CAD build for the part. Positions are in the model's coordinates, mm. Face numbers are marked on the shaded views. Give positions to 0.01 mm unless a question says otherwise; leave off trailing zeros. Loops run counter-clockwise (first coordinate to the right, second up) from the corner with the lowest first, then second, coordinate; pieces in that order, holes last. Notation, with made-up numbers: M 15,29 L 26,29 A14 ccw 26,52 Z; hole C 31,56 d6. An arc over 180 degrees is marked long. Answer as CSV lines item,"result".
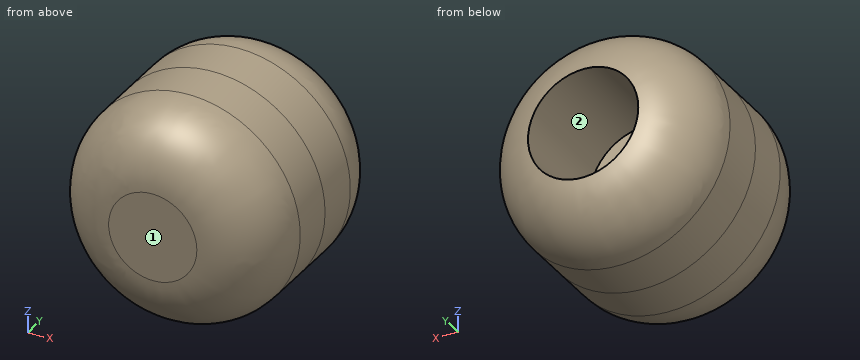
from build123d import *

# Parameters (mm, degrees)
F0_R     = 6.35
F1_DEPTH = 6.35
F2_R     = 6.35
F2_R_2   = 3.175
F3_DEPTH = 6.35


# Not quite as in the source:
# - a fillet or chamfer that OpenCascade refuses, or shapes differently, is made with other operations: its cross-section is extruded or revolved along the edge and cut away or added


with BuildPart() as f1:
    # F0 (on Front) → F1 (new body)
    with BuildSketch(Plane.XZ):
        Circle(F0_R)
    extrude(amount=F1_DEPTH)

    # F2 (on face) → F3 (join)
    with BuildSketch(Plane(origin=(0, 0, 0), x_dir=(-1, 0, 0), z_dir=(0, 1, 0))):
        Circle(F2_R)
        Circle(F2_R_2, mode=Mode.SUBTRACT)
    extrude(amount=F3_DEPTH)

    # F4: fillet of radius 3.81 on 2 edges, made by hand

    # F4_s1 → F4_t2 (revolve, cut)
    with BuildSketch(Plane.XY):
        with BuildLine():
            ThreePointArc((-6.35, 2.5932893377), (-5.4499355663, 5.0526337626), (-3.175, 6.35))
            Line((-3.175, 6.35), (-6.35, 6.35))
            Line((-6.35, 6.35), (-6.35, 2.5932893377))
        make_face()
    revolve(axis=Axis((0, 6.35, 0), (0, 1, 0)), mode=Mode.SUBTRACT)

    # F4_s3 → F4_t4 (revolve, cut)
    with BuildSketch(Plane.XY):
        with BuildLine():
            ThreePointArc((6.35, -2.54), (5.2340768363, -5.2340768363), (2.54, -6.35))
            Line((2.54, -6.35), (6.35, -6.35))
            Line((6.35, -6.35), (6.35, -2.54))
        make_face()
    revolve(axis=Axis((0, -6.35, 0), (0, -1, 0)), mode=Mode.SUBTRACT)


solid = f1.part
1) Band-saw the part on A-A on y = 1.75. Give the cut face in (x, z) (3 decimals), and give its area (3 significant figures).
Answer below:
outline,"C 0,0 d12.7; hole C 0,0 d6.35"
area,"95.0 mm^2"
2) Drill centre lines: line 1 (Z direction, x = 0, y = 1.75) (3 decimals); line 2 (Z direction, x = 5.5, y = 0.75); line 3 (Z direction, x = -2.25, y = 5.25). Where is each one in solid material? Low to high. Write a range as from..to.
Answer below:
line 1,"z = -6.35..-3.175, 3.175..6.35"
line 2,"z = -3.17..3.17"
line 3,"z = -4.77..-2.24, 2.24..4.77"
3) Mould opens along Z. For the marked faces 1 and 2 say: +Z half, -Z half, draft (parallel to the pull), parting line (faces both ways), or undercut.
Answer below:
face 1,"draft"
face 2,"undercut"
4) Band-saw the part on B-B on y = -0.25. Give the cut face in (x, z).
Answer below:
outline,"C 0,0 d12.7"
5) Flat gauge pins, fed straight in: pin 1 (1.9 mm diameter, centred on x = -1, z = 0, fed in from +Y); pin 2 (4 mm diameter, centred on y = 3, z = 2.5, fed in from +X); pin 3 (1 mm diameter, centred on x = -1, y = 2, fed in from -Z); pin 4 (7.5 mm diameter, centred on x = 0, z = 0, fed in from +Y). Where does each tip first touch, or does it go through?
Answer below:
pin 1,"stops at y = 0"
pin 2,"stops at x = 6.33"
pin 3,"stops at z = -6.33"
pin 4,"stops at y = 6.35"
